Verification items for the finished model (mm, model axes). Face numbers are marked on the shaded views. Coordinates: 2 decimals unless noted, no trailing zeros. Order: outer loops, then holes, each group sorted by start corner. A loop starts at its lowest first (then second) coordinate and runs counter-clockwise, first axis right, second up. Notation, with made-up numbers: M 41.5,-36 L 64.5,-36 A24 ccw 64.5,0 Z; hole C 20.25,-26.75 d2. An arc over 180 degrees is marked long. Return JSON: item names as keys, results as strings. Group by question number.
Q1. Thickness scan on probe 1 along Y at (x, z) = (0, 9); probe 2 along Z at (x, y) = (-18.5, -4.5); probe 3 along Z at (x, y) = (-14.5, -12). Record the ranges inside material, lowest first.
Q2. Mould release check, pull along Z, two halves, no side actions. Record for the marked faces 1, 2 and 3: pulls with the +Z half, pulls with the -Z half, needs draft (parallel to the pull), parting line crosses it, or undercut.
Q3. Section check B-B, the plane z = -29. Enter the section's corners in (x, y).
Q4. Section check A-A, the plane z = 11. Enter the section's corners in (x, y) (1 decimal), then the cut area to 3 significant figures.
Q5. Go/stop test with flat-tipped pins: pin 1 Ø10 at (y, z) = (-22.5, 25) entering from +X; pin 2 Ø3 at (x, z) = (-16.5, -1) entering from +Y; pin 3 Ø10 at (x, y) = (19.5, 24) entering from -Z; pin 4 Ø1.5 at (x, y) = (9, -26.5) entering from +Z. Record where each tip stops, or that it passes through.
from build123d import *

# Parameters (mm, degrees)
F2_R = 5.08


with BuildPart() as f1:
    # F0 (on Front) → F1 (revolve)
    with BuildSketch(Plane.XZ):
        with BuildLine():
            Line((-38.011436, -41.243773), (0, -41.243773))
            Line((0, -41.243773), (0, -35.997218))
            Line((0, -35.997218), (-29.845339, -35.997218))
            Line((-29.845339, -35.997218), (-11.164162, 0))
            Line((-11.164162, 0), (-11.164162, 46.781804))
            Line((-11.164162, 46.781804), (-16.607499, 46.781804))
            ThreePointArc((-16.607499, 46.781804), (-20.499533, 43.873593), (-16.607499, 40.965382))
            Line((-16.607499, 40.965382), (-16.607499, 0))
            Line((-16.607499, 0), (-38.011436, -41.243773))
        make_face()
    revolve(axis=Axis((0, 0, -38.620495), (0, 0, -1)))

    # F2
    f2_edges = [f1.edges().sort_by_distance(p)[0] for p in [
        (16.607499, 0, 0),
        (38.011436, 0, -41.243773),
        (-27.309468, 0, -20.621886),
        (11.164162, 0, 46.781804),
    ]]
    fillet(f2_edges, radius=F2_R)


solid = f1.part
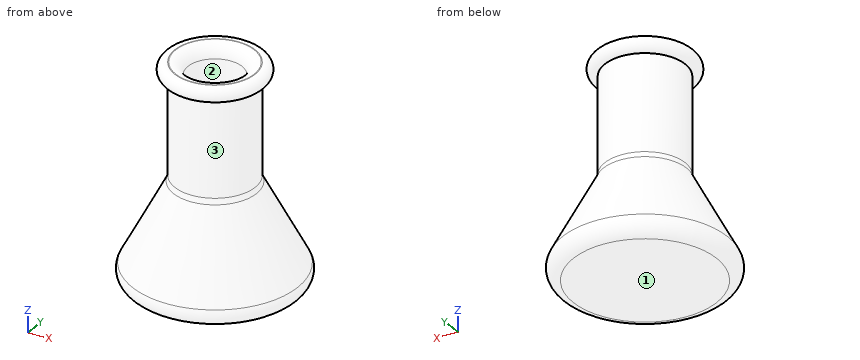
Numbers:
{
 "1": {"probe 1": "y = -16.61 to -11.16, 11.16 to 16.61", "probe 2": "z = -41.24 to -36, -15.18 to -4.69, 41.28 to 46.47", "probe 3": "z = -41.24 to -36, -14.76 to -4.27, 41.16 to 46.59"},
 "2": {"face 1": "pulls with the -Z half", "face 2": "needs draft", "face 3": "undercut"},
 "3": {"outline": "C 0,0 d63.31; hole C 0,0 d52.43"},
 "4": {"outline": "C 0,0 d33.2; hole C 0,0 d22.3", "area": "475 mm2"},
 "5": {"pin 1": "passes through", "pin 2": "stops at y = 8.7", "pin 3": "stops at z = -41.24", "pin 4": "stops at z = -20.48"}
}
